Geometry: final body of the model. Coordinates: model frame, mm. Face numbers are marked on the shaded views. A direction names the side the tool comes from. Give positions to 0.01 mm unless a question says otherwise; leave off trailing zeros. Loops run counter-clockwise (first coordinate to the right, second up) from the corner with the lowest first, then second, coordinate; pieces in that order, holes last. Notation, with made-up numbers: (18.25, 79.25) -> (67.25, 79.25) arc R30 cw to (67.25, 106.25) -> close; hole circle Ø6 at (6, 61.5). An arc over 180 degrees is marked (long way). Answer in a Markdown table with one row per item. Add a question column.
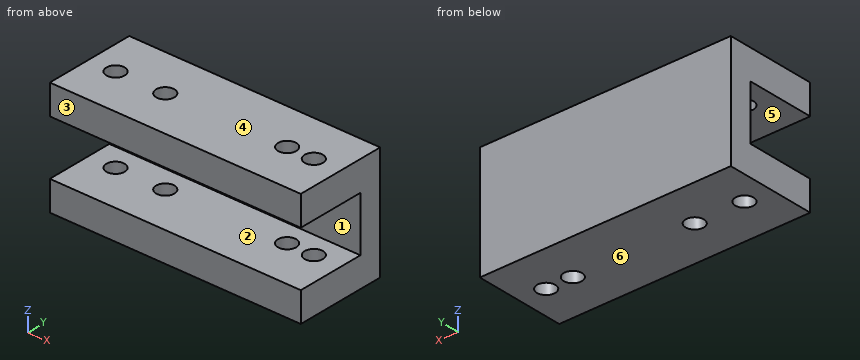
from build123d import *

# Parameters (mm, degrees)
CROQUIS4_W                 = 55
CROQUIS4_H                 = 25
SALIENTE_EXTRUIR3_DEPTH    = 20
CROQUIS5_W                 = 55
CROQUIS5_H                 = 12
CORTAR_EXTRUIR1_DEPTH      = 15
CROQUIS7_R                 = 2
CORTAR_EXTRUIR3_DEPTH      = 1
CORTAR_EXTRUIR3_DEPTH_BACK = 26
CROQUIS14_R                = 2
CORTAR_EXTRUIR6_DEPTH      = 35


with BuildPart() as part:
    # Croquis4 → Saliente-Extruir3 (new body)
    with BuildSketch(Plane(origin=(0, 0, 0), x_dir=(1, 0, 0), z_dir=(0, 1, 0))):
        with Locations((2.725806452, 3.983870968)):
            Rectangle(CROQUIS4_W, CROQUIS4_H)
    extrude(amount=SALIENTE_EXTRUIR3_DEPTH)

    # Croquis5 → Cortar-Extruir1 (cut)
    with BuildSketch(Plane(origin=(0, 0, 0), x_dir=(-1, 0, 0), z_dir=(0, -1, 0))):
        with Locations((-2.725806452, 3.983870968)):
            Rectangle(CROQUIS5_W, CROQUIS5_H)
    extrude(amount=-CORTAR_EXTRUIR1_DEPTH, mode=Mode.SUBTRACT)

    # Croquis7 → Cortar-Extruir3 (cut, two sides)
    with BuildSketch(Plane(origin=(0, 0, -16.483870968), x_dir=(-1, 0, 0), z_dir=(0, 0, -1))) as cortar_extruir3_sk:
        with Locations((-24.380806452, 10)):
            Circle(CROQUIS7_R)
        with Locations((-18.535806452, 10)):
            Circle(CROQUIS7_R)
    extrude(amount=CORTAR_EXTRUIR3_DEPTH, mode=Mode.SUBTRACT)
    extrude(cortar_extruir3_sk.sketch, amount=-CORTAR_EXTRUIR3_DEPTH_BACK, mode=Mode.SUBTRACT)

    # Croquis14 → Cortar-Extruir6 (cut)
    with BuildSketch(Plane(origin=(0, 0, -16.483870968), x_dir=(-1, 0, 0), z_dir=(0, 0, -1))):
        with Locations((8.084193548, 9.903617559)):
            Circle(CROQUIS14_R)
        with Locations((18.929193548, 9.838818962)):
            Circle(CROQUIS14_R)
    extrude(amount=-CORTAR_EXTRUIR6_DEPTH, mode=Mode.SUBTRACT)


solid = part.part
(1) Reachability of the marked faces 5 and 6 from +Z, -Z, +X, -X, +Y, -Y: full face, straight path, thin tool, end or side. Return the list, or none.
(2) Cut plane D-D on z = -2.5. Return the cut outline in (x, y), then the cut area to 3 significant figures.
(3) Cut plane C-C on x = 1. Return the cut outline in (y, z).
(4) Cut plane B-B on z = 3.25. Return the cut outline in (x, y).
(5) Draft query along Z for the marked faces 1, 2, 3 and 4. Return one class per face: +Z half, -Z half, draft (parallel to the pull), parting line (faces both ways), or undercut.
(6) Material intervals for line 1 along Z through (x, y) = (7.5, 4); line 2 along X through (y, z) = (9, 5.25); line 3 along Y through (x, z) = (-9, 1.75), sorted ascending. Write a range as from..to.
(7) Pin query (flat end, axial travel): pin 1 Ø6 at (x, z) = (0, -3.5) entering from -Y. Return the tip coordinate at first contact, or that it passes through.
(8) Cut plane A-A on y = 5.75. Return the cut outline in (x, z).
Answer list:
| question | item | result |
|---|---|---|
| 1 | face 5 | +X, -X, -Y |
| 1 | face 6 | -Z, +X, -X, +Y, -Y |
| 2 | outline | (-24.77, 15) -> (30.23, 15) -> (30.23, 20) -> (-24.77, 20) -> close |
| 2 | area | 275 mm² |
| 3 | outline | (0, -16.48) -> (20, -16.48) -> (20, 8.52) -> (0, 8.52) -> (0, 2.02) -> (15, 2.02) -> (15, -9.98) -> (0, -9.98) -> close |
| 4 | outline | (-24.77, 0) -> (30.23, 0) -> (30.23, 20) -> (-24.77, 20) -> close; hole circle Ø4 at (-18.93, 9.84); hole circle Ø4 at (-8.08, 9.9); hole circle Ø4 at (18.54, 10); hole circle Ø4 at (24.38, 10) |
| 5 | face 1 | undercut |
| 5 | face 2 | undercut |
| 5 | face 3 | draft |
| 5 | face 4 | +Z half |
| 6 | line 1 | z = -16.48..-9.98, 2.02..8.52 |
| 6 | line 2 | x = -24.77..-20.74, -17.11..-9.87, -6.3..16.8, 20.27..22.65, 26.11..30.23 |
| 6 | line 3 | y = 15..20 |
| 7 | pin 1 | stops at y = 15 |
| 8 | outline | (-24.77, -16.48) -> (30.23, -16.48) -> (30.23, -9.98) -> (-24.77, -9.98) -> close; (-24.77, 2.02) -> (30.23, 2.02) -> (30.23, 8.52) -> (-24.77, 8.52) -> close |
